Read the model definition and answer for the solid it produces. Units are mm, in the model's axes. Coordinates: 2 decimals unless noted, no trailing zeros. Order: outer loops, then holes, each group sorted by start corner. A loop starts at its lowest first (then second) coordinate and runs counter-clockwise, first axis right, second up. Notation, with made-up numbers: M -23,-23.75 L 6,-23.75 A17 ccw 6,-10.75 Z; hole C 14,66 d6. An arc over 180 degrees is marked long. Use a Markdown table: item, result. Add a question column.
1) Find the intervals of material crossed by probe 1 along Y at (x, z) = (0, -2); probe 2 along Y at (x, z) = (-38, -17); probe 3 along Y at (x, z) = (10, -11), in increasing order. Write a range as [from, to].
2) Each of these flat-tipped pins is pushed along its axis until it touches: pin 1 Ø12 at (x, z) = (-33, -4.5) entering from +Y; pin 2 Ø7.5 at (x, y) = (0, 747.13) entering from +Z; pin 3 Ø3 at (x, z) = (29.5, -11.5) entering from -Y; pin 4 Ø8 at (x, z) = (1.5, -12.5) entering from +Y. Where does it stop, or does it pass through?
3) Find section B-B on x = -32. Write down the section's boundary in (y, z), plus the area to 3 significant figures.
4) Find section A-A on z = -4. Write down the section's boundary in (x, y) (3 decimals).
from build123d import *

# Parameters (mm, degrees)
SKETCH1_W                   = 88.9
SKETCH1_H                   = 38.1
BOSS_EXTRUDE1_DEPTH         = 1016
CUT_EXTRUDE1_DEPTH          = 1018.685320961
F_1_4_0_25_DIAMETER_HOLE1_D = 6.35
FILLET1_R                   = 3.175


with BuildPart() as part:
    # Sketch1 → Boss-Extrude1 (new body)
    with BuildSketch(Plane(origin=(0, 0, 0), x_dir=(1, 0, 0), z_dir=(0, 1, 0))):
        Rectangle(SKETCH1_W, SKETCH1_H)
    extrude(amount=BOSS_EXTRUDE1_DEPTH)

    # Sketch2 → Cut-Extrude1 (cut, through all)
    with BuildSketch(Plane.XY.offset(19.05)):
        Polygon((44.45, 0), (-44.45, 0), (-44.45, 15.675468585), align=None)
        Polygon((-44.45, 1016), (44.45, 1000.324531415), (44.45, 1016), align=None)
    extrude(amount=-CUT_EXTRUDE1_DEPTH, mode=Mode.SUBTRACT)

    # 1/4 (0.25) Diameter Hole1 (through all)
    with Locations(Plane.XY.offset(19.05)):
        with Locations((18.786968779, 68.737585765), (0, 187.400991466), (0, 747.126552809), (0, 963.026552809)):
            Hole(F_1_4_0_25_DIAMETER_HOLE1_D / 2)

    # Fillet1
    fillet1_edges = [part.edges().sort_by_distance(p)[0] for p in [
        (44.45, 500.162265708, -19.05),
        (44.45, 500.162265708, 19.05),
        (-44.45, 515.837734292, -19.05),
        (-44.45, 515.837734292, 19.05),
    ]]
    fillet(fillet1_edges, radius=FILLET1_R)


solid = part.part
Check result:
| question | item | result |
|---|---|---|
| 1 | probe 1 | y = [7.84, 184.23], [190.58, 743.95], [750.3, 959.85], [966.2, 1008.16] |
| 1 | probe 2 | y = [14.54, 1014.86] |
| 1 | probe 3 | y = [6.07, 1006.4] |
| 2 | pin 1 | stops at y = 1015.04 |
| 2 | pin 2 | stops at z = 19.05 |
| 2 | pin 3 | stops at y = 2.37 |
| 2 | pin 4 | stops at y = 1008.6 |
| 3 | outline | M 13.48,-19.05 L 1013.8,-19.05 L 1013.8,19.05 L 13.48,19.05 Z |
| 3 | area | 38,100 mm2 |
| 4 | outline | M -44.45,15.675 L 44.45,0 L 44.45,1000.325 L -44.45,1016 Z; hole C 0,187.401 d6.35; hole C 0,747.127 d6.35; hole C 0,963.027 d6.35; hole C 18.787,68.738 d6.35 |
